Read the model definition and answer for the solid it produces. Units are mm, in the model's axes. Face numbers are marked on the shaded views. A direction names the side the tool comes from. Coordinates: 2 decimals unless noted, no trailing zeros. Write each loop counter-clockwise with the first axis right and the second up, starting at its lowest first coordinate (ties: lowest second). Pieces come first, ordered by that corner, then holes.
1) Determine the mould class of the marked faces 4, 5 and 6 for opening direction Y: +Y half, -Y half, draft (parallel to the pull), parting line (faces both ways), or undercut.
2) Each of these flat-tipped pins is pushed along its axis until it touches: pin 1 Ø0.9 at (x, y) = (14.5, 98.5) entering from -Z; pin 2 Ø11 at (x, y) = (-1.5, 57) entering from +Z; pin 3 Ø5 at (y, z) = (85.5, -7.5) entering from -X; pin 4 Ø7 at (y, z) = (69, 1.5) entering from +X. Where does it stop, or does it pass through?
3) Which of the six approach directions +Z, -Z, +X, -X, +Y, -Y give full straight-line access (tool end or side, diameter ignored) to the marked faces 1, 2 and 3?
4) The part is cut by section C-C (y = 26). Determine the outline of the cut face in (x, z), then the cut area to 3 significant figures.
5) The part is cut by section D-D (x = -23.5). Determine the outline of the cut face in (y, z), then the cut area to 3 significant figures.
6) The part is cut by section B-B (x = 0). Determine the outline of the cut face in (y, z).
7) Find the intervals of material crossed by line 1 (X direction, y = 98.85, z = 6); line 2 (X direction, y = 18.5, z = -4); line 3 (Z direction, x = 17.5, y = 98.05), in increasing order.
8) The part is cut by section A-A (z = -2). Determine the outline of the cut face in (x, y).
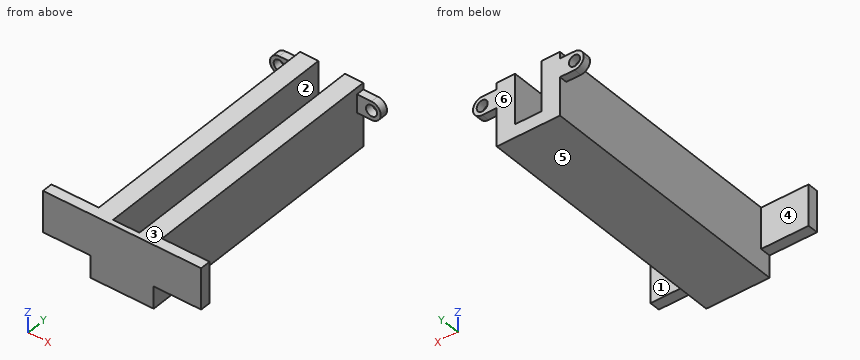
from build123d import *

# Parameters (mm, degrees)
SKETCH1_W            = 24
SKETCH1_H            = 24
BOSS_EXTRUDE1_DEPTH  = 100
SKETCH3_W            = 10
SKETCH3_H            = 19
CUT_EXTRUDE1_DEPTH   = 98
SKETCH6_W            = 24
SKETCH6_H            = 4
BOSS_EXTRUDE3_DEPTH  = 18
SKETCH7_W            = 18
SKETCH7_H            = 8.4
CUT_EXTRUDE3_DEPTH   = 4
SKETCH8_R            = 4
CUT_EXTRUDE4_DEPTH   = 1
SKETCH9_W            = 9
SKETCH9_H            = 7
BOSS_EXTRUDE4_DEPTH  = 3
FILLET1_R            = 3.5
SKETCH10_R           = 2.1
CUT_EXTRUDE5_DEPTH   = 3
FILLET1_OF_MIRROR3_R = 3.5


with BuildPart() as part:
    # Sketch1 → Boss-Extrude1 (new body)
    with BuildSketch(Plane(origin=(0, 0, 0), x_dir=(1, 0, 0), z_dir=(0, 1, 0))):
        Rectangle(SKETCH1_W, SKETCH1_H)
    extrude(amount=BOSS_EXTRUDE1_DEPTH)

    # Sketch3 → Cut-Extrude1 (cut)
    with BuildSketch(Plane(origin=(0, 100, 0), x_dir=(1, 0, 0), z_dir=(0, 1, 0))):
        with Locations((0, -2.5)):
            Rectangle(SKETCH3_W, SKETCH3_H)
    extrude(amount=-CUT_EXTRUDE1_DEPTH, mode=Mode.SUBTRACT)

    # Sketch6 → Boss-Extrude3 (add)
    with BuildSketch(Plane.ZY.offset(12)):
        with Locations((0, 2)):
            Rectangle(SKETCH6_W, SKETCH6_H)
    boss_extrude3 = extrude(amount=BOSS_EXTRUDE3_DEPTH)

    # Sketch7 → Cut-Extrude3 (cut)
    with BuildSketch(Plane(origin=(0, 4, 0), x_dir=(1, 0, 0), z_dir=(0, 1, 0))):
        with Locations((-21, 7.8)):
            Rectangle(SKETCH7_W, SKETCH7_H)
    cut_extrude3 = extrude(amount=-CUT_EXTRUDE3_DEPTH, mode=Mode.SUBTRACT)

    # Mirror2: Boss-Extrude3, Cut-Extrude3 across plane
    add(boss_extrude3.mirror(Plane(origin=(0, 0, 0), x_dir=(0, 0, 1), z_dir=(1, 0, 0))))
    add(cut_extrude3.mirror(Plane(origin=(0, 0, 0), x_dir=(0, 0, 1), z_dir=(1, 0, 0))), mode=Mode.SUBTRACT)

    # Sketch8 → Cut-Extrude4 (cut)
    with BuildSketch(Plane(origin=(0, 2, 0), x_dir=(1, 0, 0), z_dir=(0, 1, 0))):
        with Locations(Location((0, 2, 0), (0, 0, 270))):
            Circle(SKETCH8_R)
    extrude(amount=-CUT_EXTRUDE4_DEPTH, mode=Mode.SUBTRACT)

    # Sketch9 → Boss-Extrude4 (add)
    with BuildSketch(Plane(origin=(0, 100, 0), x_dir=(1, 0, 0), z_dir=(0, 1, 0))):
        with Locations((-16.5, -6)):
            Rectangle(SKETCH9_W, SKETCH9_H)
    boss_extrude4 = extrude(amount=-BOSS_EXTRUDE4_DEPTH)

    # Fillet1
    fillet1_edges = [part.edges().sort_by_distance(p)[0] for p in [
        (-21, 98.5, 2.5),
        (-21, 98.5, 9.5),
    ]]
    fillet(fillet1_edges, radius=FILLET1_R - 0.0001)  # a hair under: the kernel refuses the full size

    # Sketch10 → Cut-Extrude5 (cut)
    with BuildSketch(Plane(origin=(0, 100, 0), x_dir=(1, 0, 0), z_dir=(0, 1, 0))):
        with Locations(Location((-17.5, -6, 0), (0, 0, 270))):
            Circle(SKETCH10_R)
    cut_extrude5 = extrude(amount=-CUT_EXTRUDE5_DEPTH, mode=Mode.SUBTRACT)

    # Mirror3: Boss-Extrude4, Cut-Extrude5 across plane
    add(boss_extrude4.mirror(Plane(origin=(0, 0, 0), x_dir=(0, 0, 1), z_dir=(1, 0, 0))))
    add(cut_extrude5.mirror(Plane(origin=(0, 0, 0), x_dir=(0, 0, 1), z_dir=(1, 0, 0))), mode=Mode.SUBTRACT)

    # Fillet1 of Mirror3
    fillet1_of_mirror3_edges = [part.edges().sort_by_distance(p)[0] for p in [
        (21, 98.5, 2.5),
        (21, 98.5, 9.5),
    ]]
    fillet(fillet1_of_mirror3_edges, radius=FILLET1_OF_MIRROR3_R - 0.0001)  # a hair under: the kernel refuses the full size


solid = part.part
Reported:
1. face 4: undercut
1. face 5: draft
1. face 6: +Y half
2. pin 1: stops at z = 2.5
2. pin 2: stops at z = 12
2. pin 3: stops at x = -12
2. pin 4: stops at x = 12
3. face 1: +Z, -Z, +X
3. face 2: +Z, +Y
3. face 3: +Z, +X, -X, +Y, -Y
4. outline: (-12, -12) - (12, -12) - (12, 12) - (5, 12) - (5, -7) - (-5, -7) - (-5, 12) - (-12, 12) - close
4. area: 386 mm2
5. outline: (0, -3.6) - (4, -3.6) - (4, 12) - (0, 12) - close
5. area: 62.4 mm2
6. outline: (0, -12) - (100, -12) - (100, -7) - (2, -7) - (2, -6) - (1, -6) - (1, 2) - (2, 2) - (2, 12) - (0, 12) - close
7. line 1: x = -21 to -19.6, -15.4 to -5, 5 to 15.4, 19.6 to 21
7. line 2: x = -12 to -5, 5 to 12
7. line 3: z = 2.5 to 3.9, 8.1 to 9.5
8. outline: (-30, 0) - (30, 0) - (30, 4) - (12, 4) - (12, 100) - (5, 100) - (5, 2) - (4, 2) - (4, 1) - (-4, 1) - (-4, 2) - (-5, 2) - (-5, 100) - (-12, 100) - (-12, 4) - (-30, 4) - close
